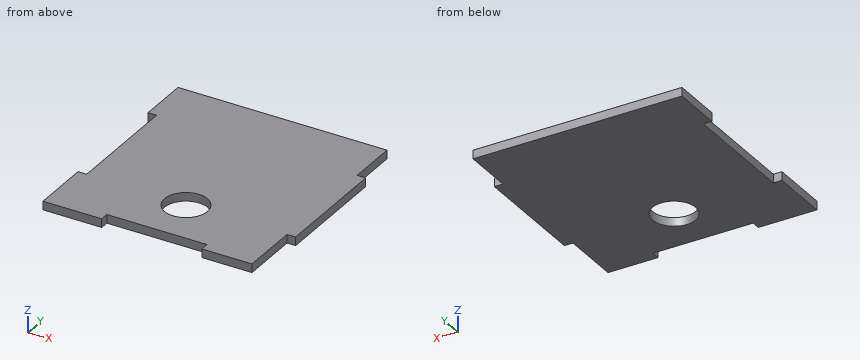
from build123d import *

# Parameters (mm, degrees)
BOSS_EXTRUDE1_DEPTH = 3
SKETCH2_R           = 7.5
CUT_EXTRUDE1_DEPTH  = 3


with BuildPart() as part:
    # Sketch1 → Boss-Extrude1 (new body)
    with BuildSketch(Plane.XY):
        Polygon((-35, 38), (-17.5, 38), (17.5, 38), (35, 38), (35, 20.5), (38, 20.5), (38, -20.5), (35, -20.5), (35, -38), (35, -41), (17.5, -41), (17.5, -38), (-17.5, -38), (-17.5, -41), (-35, -41), (-38, -41), (-38, -38), (-38, -20.5), (-35, -20.5), (-35, 20.5), (-38, 20.5), (-38, 38), align=None)
    extrude(amount=BOSS_EXTRUDE1_DEPTH)

    # Sketch2 → Cut-Extrude1 (cut)
    with BuildSketch(Plane.XY.offset(3)):
        with Locations((0, -21)):
            Circle(SKETCH2_R)
    extrude(amount=-CUT_EXTRUDE1_DEPTH, mode=Mode.SUBTRACT)


solid = part.part
CAD build for the part. Positions are in the model's coordinates, mm. Give positions to 0.01 mm unless a question says otherwise; leave off trailing zeros. Order: outer loops, then holes, each group sorted by start corner. A loop starts at its lowest first (then second) coordinate and runs counter-clockwise, first axis right, second up. Notation, with made-up numbers: (73, 17) - (78, 17) arc R34 cw to (78, 47) - close; hole circle Ø9 at (6.25, -17.75). An arc over 180 degrees is marked (long way). Write each question's results on one line, items separated by ' | '.
1. Saw through at C-C on z = 0.45. List the corners of the cut face in (x, y), and give its area (3 significant figures).
Calculated:
outline: (-38, -41) - (-17.5, -41) - (-17.5, -38) - (17.5, -38) - (17.5, -41) - (35, -41) - (35, -20.5) - (38, -20.5) - (38, 20.5) - (35, 20.5) - (35, 38) - (-38, 38) - (-38, 20.5) - (-35, 20.5) - (-35, -20.5) - (-38, -20.5) - close; hole circle Ø15 at (0, -21) | area: 5,490 mm2
2. Saw through at B-B on y = -27. List the corners of the cut face in (x, z).
Calculated:
outline: (-38, 0) - (-4.5, 0) - (-4.5, 3) - (-38, 3) - close; (4.5, 0) - (35, 0) - (35, 3) - (4.5, 3) - close
3. Probe L1, parallel to Y at x = 0, z = 0.9; L2, parallel to X at y = 19.5, z = 1.2; L3, parallel to X at y = -32.5, z = 2.4. List the from-to ranges inside material, lowest first. Write a range as from..to.
Calculated:
L1: y = -38..-28.5, -13.5..38 | L2: x = -35..38 | L3: x = -38..35
4. Pin check, flat tip, straight feed: pin 1 (1.5 mm diameter, centred on y = -30, z = 2, fed in from +X). Stop position of the tip, or through.
Calculated:
pin 1: stops at x = 35
5. Saw through at D-D on x = 9.5. List the corners of the cut face in (y, z).
Calculated:
outline: (-38, 0) - (38, 0) - (38, 3) - (-38, 3) - close
6. Saw through at A-A on x = 0. List the corners of the cut face in (y, z).
Calculated:
outline: (-38, 0) - (-28.5, 0) - (-28.5, 3) - (-38, 3) - close; (-13.5, 0) - (38, 0) - (38, 3) - (-13.5, 3) - close
